from build123d import *

# Parameters (mm, degrees)
SKETCH1_W           = 20
SKETCH1_H           = 27.6
BOSS_EXTRUDE1_DEPTH = 4
SKETCH3_R           = 1
CUT_EXTRUDE2_DEPTH  = 4
SKETCH4_W           = 1.6
SKETCH4_H           = 3
SKETCH4_W_2         = 1.8
SKETCH4_H_2         = 4.5
CUT_EXTRUDE3_DEPTH  = 25.626002518
CUT_EXTRUDE4_REACH  = 20.827
SKETCH5_R           = 1.5
SKETCH6_R           = 1
CUT_EXTRUDE5_DEPTH  = 1
SKETCH7_R           = 0.6
CUT_EXTRUDE6_DEPTH  = 30.627014699
FILLET1_R           = 1
FILLET2_R           = 0.2


with BuildPart() as part:
    # Sketch1 → Boss-Extrude1 (new, symmetric)
    with BuildSketch(Plane.XY):
        Rectangle(SKETCH1_W, SKETCH1_H)
    extrude(amount=BOSS_EXTRUDE1_DEPTH, both=True)

    # Sketch3 → Cut-Extrude2 (cut)
    with BuildSketch(Plane.XY.offset(4)):
        with Locations((-5, 0)):
            Circle(SKETCH3_R)
    extrude(amount=-CUT_EXTRUDE2_DEPTH, mode=Mode.SUBTRACT)

    # Sketch4 → Cut-Extrude3 (cut, through all)
    with BuildSketch(Plane(origin=(10, 0, 0), x_dir=(0, 0, -1), z_dir=(1, 0, 0))):
        with Locations((3.2, 8.5)):
            Rectangle(SKETCH4_W, SKETCH4_H)
        with Locations((1.5, 8.5)):
            Rectangle(SKETCH4_W_2, SKETCH4_H_2)
    cut_extrude3 = extrude(amount=-CUT_EXTRUDE3_DEPTH, mode=Mode.SUBTRACT)

    # Cut-Extrude4: up to this face of the body (flat: up to its plane)
    cut_extrude4_end = Plane(part.part.faces().sort_by_distance((0, 8.5, -0.6))[0])
    # Sketch5 → Cut-Extrude4 (cut, up to the picked face)
    with BuildSketch(Plane(origin=(0, 0, -4), x_dir=(-1, 0, 0), z_dir=(0, 0, -1)), mode=Mode.PRIVATE) as cut_extrude4_sk1:
        with Locations((0, 7)):
            Circle(SKETCH5_R)
    cut_extrude4_tool1 = split(extrude(cut_extrude4_sk1.sketch, amount=-CUT_EXTRUDE4_REACH, mode=Mode.PRIVATE), bisect_by=cut_extrude4_end, keep=Keep.BOTH, mode=Mode.PRIVATE)
    cut_extrude4 = cut_extrude4_tool1.solids().sort_by(Axis((0, 7, -4), (0, 0, 1)))[0]
    add(cut_extrude4, mode=Mode.SUBTRACT)

    # Mirror1: Cut-Extrude3, Cut-Extrude4 across plane
    add(cut_extrude3.mirror(Plane.ZX), mode=Mode.SUBTRACT)
    add(cut_extrude4.mirror(Plane.ZX), mode=Mode.SUBTRACT)

    # Sketch6 → Cut-Extrude5 (cut)
    with BuildSketch(Plane.XZ.offset(13.8)):
        with Locations((-7, -1.5)):
            Circle(SKETCH6_R)
        with Locations(Location((7, -1.5, 0), (0, 0, 180))):
            Circle(SKETCH6_R)
    cut_extrude5 = extrude(amount=-CUT_EXTRUDE5_DEPTH, mode=Mode.SUBTRACT)

    # Sketch7 → Cut-Extrude6 (cut, through all)
    with BuildSketch(Plane.XZ.offset(13.8)):
        with Locations((-7, -1.5)):
            Circle(SKETCH7_R)
        with Locations((7, -1.5)):
            Circle(SKETCH7_R)
    extrude(amount=-CUT_EXTRUDE6_DEPTH, mode=Mode.SUBTRACT)

    # Fillet1
    fillet1_edges = [part.edges().sort_by_distance(p)[0] for p in [
        (-1.5, 7, -3.2),
        (1.5, 7, -3.2),
        (1.5, -7, -3.2),
        (-1.5, -7, -3.2),
    ]]
    fillet(fillet1_edges, radius=FILLET1_R)

    # Mirror2: Cut-Extrude5 across plane
    add(cut_extrude5.mirror(Plane.ZX), mode=Mode.SUBTRACT)

    # Fillet2
    fillet2_edges = [part.edges().sort_by_distance(p)[0] for p in [
        (-8, -13.8, -1.5),
        (8, -13.8, -1.5),
        (0, 13.8, 4),
        (-8, 13.8, -1.5),
        (8, 13.8, -1.5),
        (0, 13.8, -4),
        (0, -13.8, -4),
        (0, -13.8, 4),
    ]]
    fillet(fillet2_edges, radius=FILLET2_R)


solid = part.part
For this review, take the finished solid that the model builds, in its own axes (mm). A direction names the side the tool comes from. Round coordinates to 2 decimals unless told otherwise and drop trailing zeros. Loops run counter-clockwise (first coordinate to the right, second up) from the corner with the lowest first, then second, coordinate; pieces in that order, holes last. Notation, with made-up numbers: (86.25, 53.25) - (120.25, 53.25) arc R13 cw to (120.25, 72.25) - close; hole circle Ø10 at (4, 54.5). An arc over 180 degrees is marked (long way). Put each result on its own line as item: value. Start each with the question number.
1. Consider section D-D on x = -7. State how many separate pieces and enclosed holes the cut face has, plus the area to 3 significant figures.
2. Consider section B-B on x = -5. State the section outline as (y, z) points, plus the area to 3 significant figures.
3. Consider section A-A on z = -3. State the section outline as (x, y) points, plus the area to 3 significant figures.
4. Consider section C-C on y = 0. State the section outline as (x, z) points.
5. For faces 4 (the flat face through (-5, 0, 0)), 5 (the cylindrical face through (-1.75, 6.84, -3.19)), 6 (the flat face through (0, -10.75, -1)), 7 (the flat face through (6, 7, -3)), list the 3-axis set-ups (+Z, -Z, +X, -X, +Y, -Y) from which the entire face can be reached by the end or side of a thin tool; tool diameter is ignored.
6. Insertion check: P1, Ø1.4, axis at x = -7, z = -1.5, coming from the -Y side. The pin has a flat end and moves straight along its axis. Give the tip position at first contact, or say it passes through.
7. Mouldability with a two-part tool opening along Y and no side actions: class faces 1 (the flat face through (0, -13.8, 0)), 2 (the flat face through (6, 6.25, -1)), 3 (the cylindrical face through (-7.217, 13.206, -2.476)) as +Y half, -Y half, draft (parallel to the pull), parting line (faces both ways), or undercut.
8. For probe 1 along Y at (x, z) = (4, -3.25); probe 2 along Y at (x, z) = (-3, -1.25); probe 3 along Z at (x, y) = (7, -12.1), list the stretches that pass through material, from the lowest coordinate up. Write a range as [from, to].
Result sheet:
1. separate pieces: 4
1. enclosed holes: 0
1. area: 171 mm^2
2. outline: (-13.8, -3.8) arc R0.2 ccw to (-13.6, -4) - (-10, -4) - (-10, -2.4) - (-10.75, -2.4) - (-10.75, -0.6) - (-6.25, -0.6) - (-6.25, -2.4) - (-7, -2.4) - (-7, -4) - (7, -4) - (7, -2.4) - (6.25, -2.4) - (6.25, -0.6) - (10.75, -0.6) - (10.75, -2.4) - (10, -2.4) - (10, -4) - (13.6, -4) arc R0.2 ccw to (13.8, -3.8) - (13.8, 3.8) arc R0.2 ccw to (13.6, 4) - (1, 4) - (1, 0) - (-1, 0) - (-1, 4) - (-13.6, 4) arc R0.2 ccw to (-13.8, 3.8) - close
2. area: 187 mm^2
3. outline: (-10, -13.8) - (10, -13.8) - (10, -10) - (-10, -10) - close; (-10, -7) - (-2.29, -7) arc R1 ccw to (-1.37, -6.4) arc R1.5 cw to (1.37, -6.4) arc R1 ccw to (2.29, -7) - (10, -7) - (10, 7) - (2.29, 7) arc R1 ccw to (1.37, 6.4) arc R1.5 cw to (-1.37, 6.4) arc R1 ccw to (-2.29, 7) - (-10, 7) - close; (-10, 10) - (10, 10) - (10, 13.8) - (-10, 13.8) - close
3. area: 425 mm^2
4. outline: (-10, -4) - (10, -4) - (10, 4) - (-4, 4) - (-4, 0) - (-6, 0) - (-6, 4) - (-10, 4) - close; hole circle Ø1.2 at (-7, -1.5); hole circle Ø1.2 at (7, -1.5)
5. face 4: +Z
5. face 5: -Z
5. face 6: +X, -X
5. face 7: -Z, +X, -X
6. P1: y = -12.8
7. face 1: -Y half
7. face 2: undercut
7. face 3: draft
8. probe 1: [-13.8, -10], [-7, 7], [10, 13.8]
8. probe 2: [-13.8, -10.75], [-6.25, 6.25], [10.75, 13.8]
8. probe 3: [-4, -2.1], [-0.9, 4]
